Input: part model. Units: mm. Frame: model coordinates. A direction names the side the tool comes from. Give positions to 0.01 mm unless a question says otherwise; leave off trailing zeros. Write each loop counter-clockwise with the first axis right and the second up, starting at its lowest first coordinate (ties: lowest second). Pieces come first, ordered by that corner, then holes. Notation, with made-up numbers: (53, 23) - (106, 23) arc R32 cw to (106, 49) - close; hole circle Ø7 at (23, 21.25). An arc over 180 degrees is marked (long way). Use a Markdown table: item, result. Add a question column.
1. Section query D-D, the plane y = -4.4. Return loops of the section in (x, z).
2. Pin query (flat end, axial travel): pin 1 (2.5 mm diameter, centred on x = 0, z = 11, fed in from +Y); pin 2 (2.5 mm diameter, centred on x = 0, y = -3.5, fed in from +Z). Return the tip coordinate at first contact, or that it passes through.
3. Section query C-C, the plane x = -11. Return loops of the section in (y, z), plus the area to 3 significant figures.
4. Mould query, pull axis Z, two halves, no side actions, for faces 1 (the cylindrical face through (-0.325, -2.465, 9.536)), 2 (the flat face through (0, -2, 22.5)), 3 (the cylindrical face through (9.5, -2.46, 0.07)), 4 (the flat face through (5, -2, 25)). Classes: released by +Z, released by -Z, zero draft, split by the parting line, or undercut.
5. Section query B-B, the plane x = 0. Return loops of the section in (y, z).
6. Set-up query: faces 5 (the flat face through (-15, -2, 27.5)), 6 (the flat face through (-5, -2, 25)). Return all of +Z, -Z, +X, -X, +Y, -Y with unobstructed straight access to the full face (end or side cutting, diameter ignored); none if empty.
7. Material intervals for probe 1 along Z at (x, y) = (0, -4.7); probe 2 along Z at (x, y) = (11, -1.7); probe 3 along Z at (x, y) = (-12, -1.4), sorted ascending.
8. Section query A-A, the plane z = 0. Return loops of the section in (x, y), plus the area to 3 significant figures.
```python
from build123d import *

# Parameters (mm, degrees)
F0_R     = 1.5
F0_R_2   = 2.5
F0_R_3   = 5
F1_DEPTH = 5


with BuildPart() as f1:
    # F0 (on Front) → F1 (new body)
    with BuildSketch(Plane.XZ):
        Polygon((25, -27.5), (25, 27.5), (5, 27.5), (5, 22.5), (-5, 22.5), (-5, 27.5), (-25, 27.5), (-25, -27.5), (-17.784204334, -27.5), (-7.784204334, -27.5), align=None)
        with Locations((0, -11)):
            Circle(F0_R, mode=Mode.SUBTRACT)
        with Locations((-11, 0)):
            Circle(F0_R, mode=Mode.SUBTRACT)
        with Locations((-12.5, 23.8740361482)):
            Circle(F0_R_2, mode=Mode.SUBTRACT)
        Circle(F0_R_3, mode=Mode.SUBTRACT)
        with Locations((11, 0)):
            Circle(F0_R, mode=Mode.SUBTRACT)
        with Locations((0, 11)):
            Circle(F0_R, mode=Mode.SUBTRACT)
        with Locations((12.5, 23.8740361482)):
            Circle(F0_R_2, mode=Mode.SUBTRACT)
    extrude(amount=F1_DEPTH)


solid = f1.part
```
Result sheet:
| question | item | result |
|---|---|---|
| 1 | outline | (-25, -27.5) - (25, -27.5) - (25, 27.5) - (5, 27.5) - (5, 22.5) - (-5, 22.5) - (-5, 27.5) - (-25, 27.5) - close; hole circle Ø5 at (-12.5, 23.87); hole circle Ø3 at (-11, 0); hole circle Ø10 at (0, 0); hole circle Ø3 at (0, -11); hole circle Ø3 at (0, 11); hole circle Ø3 at (11, 0); hole circle Ø5 at (12.5, 23.87) |
| 2 | pin 1 | passes through |
| 2 | pin 2 | stops at z = 22.5 |
| 3 | outline | (-5, -27.5) - (0, -27.5) - (0, -1.5) - (-5, -1.5) - close; (-5, 1.5) - (0, 1.5) - (0, 21.87) - (-5, 21.87) - close; (-5, 25.87) - (0, 25.87) - (0, 27.5) - (-5, 27.5) - close |
| 3 | area | 240 mm² |
| 4 | face 1 | undercut |
| 4 | face 2 | released by +Z |
| 4 | face 3 | undercut |
| 4 | face 4 | zero draft |
| 5 | outline | (-5, -27.5) - (0, -27.5) - (0, -12.5) - (-5, -12.5) - close; (-5, -9.5) - (0, -9.5) - (0, -5) - (-5, -5) - close; (-5, 5) - (0, 5) - (0, 9.5) - (-5, 9.5) - close; (-5, 12.5) - (0, 12.5) - (0, 22.5) - (-5, 22.5) - close |
| 6 | face 5 | +Z, +X, -X, +Y, -Y |
| 6 | face 6 | +Z, +Y, -Y |
| 7 | probe 1 | z = -27.5 to -12.5, -9.5 to -5, 5 to 9.5, 12.5 to 22.5 |
| 7 | probe 2 | z = -27.5 to -1.5, 1.5 to 21.87, 25.87 to 27.5 |
| 7 | probe 3 | z = -27.5 to -1.12, 1.12 to 21.42, 26.32 to 27.5 |
| 8 | outline | (-25, -5) - (-12.5, -5) - (-12.5, 0) - (-25, 0) - close; (-9.5, -5) - (-5, -5) - (-5, 0) - (-9.5, 0) - close; (5, -5) - (9.5, -5) - (9.5, 0) - (5, 0) - close; (12.5, -5) - (25, -5) - (25, 0) - (12.5, 0) - close |
| 8 | area | 170 mm² |
